Read the model definition and answer for the solid it produces. Units are mm, in the model's axes. Face numbers are marked on the shaded views. A direction names the side the tool comes from. Give positions to 0.01 mm unless a question says otherwise; leave off trailing zeros. Write each loop counter-clockwise with the first axis right and the second up, starting at its lowest first coordinate (ties: lowest second). Pieces come first, ordered by that corner, then holes. Notation, with made-up numbers: (38.5, 19.5) -> (58.5, 19.5) arc R10 cw to (58.5, 38.5) -> close; hole circle Ø11 at (-16.75, 22.25). An arc over 180 degrees is marked (long way). Use a Markdown table: item, result.
from build123d import *

# Parameters (mm, degrees)
EXTRUDE_THIN1_DEPTH     = 31.75
CUT_EXTRUDE1_DEPTH      = 79.232951004
CUT_EXTRUDE1_DEPTH_BACK = 79.232951004
SKETCH2_R               = 4.7625
SKETCH3_R               = 3.175
CUT_EXTRUDE2_DEPTH      = 56.93322439
FILLET1_R               = 9.525


with BuildPart() as part:
    # Sketch1 → Extrude-Thin1 (new, symmetric)
    with BuildSketch(Plane(origin=(0, 0, 0), x_dir=(0, 0, -1), z_dir=(1, 0, 0))):
        Polygon((0, 19.05), (0, 0), (-7.385338648, -15.83790984), (-10.372239485, -44.256373), (-12.721499107, -44.009455864), (-9.693278511, -15.19786147), (-2.3622, 0.523687132), (-2.3622, 19.05), align=None)
    extrude(amount=EXTRUDE_THIN1_DEPTH, both=True)

    # Sketch2 → Cut-Extrude1 (cut, two sides: drawn at the far end of the back side and taken through both)
    with BuildSketch(Plane(origin=(0, -51.169527341, 13.474052944), x_dir=(-1, 0, 0), z_dir=(0, 0.10452846326765357, 0.9945218953682734)).offset(-CUT_EXTRUDE1_DEPTH_BACK)):
        with Locations(Location((0, -26.249511152, 0), (0, 0, 270))):
            Circle(SKETCH2_R)
    extrude(amount=CUT_EXTRUDE1_DEPTH + CUT_EXTRUDE1_DEPTH_BACK, mode=Mode.SUBTRACT)

    # Sketch3 → Cut-Extrude2 (cut, through all)
    with BuildSketch(Plane(origin=(0, 0, 0), x_dir=(-1, 0, 0), z_dir=(0, 0, -1))):
        with Locations(Location((-22.225, 9.525, 0), (0, 0, 90))):
            Circle(SKETCH3_R)
        with Locations(Location((22.225, 9.525, 0), (0, 0, 90))):
            Circle(SKETCH3_R)
    extrude(amount=-CUT_EXTRUDE2_DEPTH, mode=Mode.SUBTRACT)

    # Fillet1
    fillet1_edges = [part.edges().sort_by_distance(p)[0] for p in [
        (31.75, 19.05, 1.1811),
        (-31.75, 19.05, 1.1811),
        (31.75, -44.132914432, 11.546869296),
        (-31.75, -44.132914432, 11.546869296),
    ]]
    fillet(fillet1_edges, radius=FILLET1_R)


solid = part.part
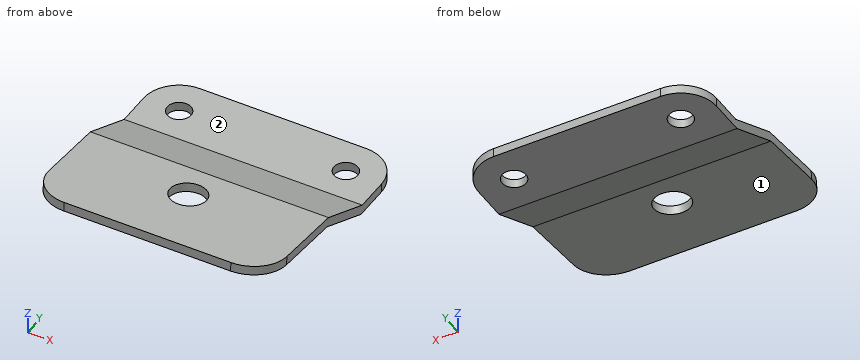
Item 1: A cutting plane is placed at D-D (x = 24.5). Give the vertices of the cut face in (y, z), then the cut area to 3 significant figures.
Return value:
| item | result |
|---|---|
| outline | (-43.98, 10.34) -> (-15.84, 7.39) -> (0, 0) -> (7.31, 0) -> (7.31, 2.36) -> (0.52, 2.36) -> (-15.2, 9.69) -> (-43.74, 12.69) -> close; (11.74, 0) -> (18.77, 0) -> (18.77, 2.36) -> (11.74, 2.36) -> close |
| area | 142 mm^2 |
Item 2: Straight lines are drawn through the part: line 1 along Z through (x, y) = (-8, 5); line 2 along X through (y, z) = (-28, 11); line 3 along Y through (x, z) = (-22, 1.5). For each, find the intervals that lie inside material, in ascending order. Write a range as [from, to].
Return value:
| item | result |
|---|---|
| line 1 | [0, 2.36] |
| line 2 | [-31.75, -3.74], [3.74, 31.75] |
| line 3 | [-3.22, 6.36], [12.69, 19.05] |
Item 3: A tool of negligible diameter and unlimited length cuts with its end or side. For the marked faces 1 and 2, from which of +Z, -Z, +X, -X, +Y, -Y can it reach the whole face along a straight path? Write none if from no direction.
Return value:
| item | result |
|---|---|
| face 1 | -Z, +X, -X, -Y |
| face 2 | +Z, +X, -X, +Y |
Item 4: A cutting plane is placed at C-C (x = -14.5). Give the vertices of the cut face in (y, z), then the cut area to 3 significant figures.
Return value:
| item | result |
|---|---|
| outline | (-44.26, 10.37) -> (-15.84, 7.39) -> (0, 0) -> (19.05, 0) -> (19.05, 2.36) -> (0.52, 2.36) -> (-15.2, 9.69) -> (-44.01, 12.72) -> close |
| area | 153 mm^2 |
Item 5: A cutting plane is placed at B-B (z = 1). Count the separate pieces of the cut face and the enclosed holes in it, then the cut area to 3 significant figures.
Return value:
| item | result |
|---|---|
| separate pieces | 1 |
| enclosed holes | 2 |
| area | 1,240 mm^2 |
Item 6: A cutting plane is placed at A-A (x = 3). Give the vertices of the cut face in (y, z), then the cut area to 3 significant figures.
Return value:
| item | result |
|---|---|
| outline | (-44.26, 10.37) -> (-28.99, 8.77) -> (-28.74, 11.12) -> (-44.01, 12.72) -> close; (-21.63, 7.99) -> (-15.84, 7.39) -> (0, 0) -> (19.05, 0) -> (19.05, 2.36) -> (0.52, 2.36) -> (-15.2, 9.69) -> (-21.39, 10.34) -> close |
| area | 136 mm^2 |
Item 7: Each of these flat-tipped pins is pushed along its axis until it touches: P1, Ø7.5, axis at x = -22.225, y = 9.525, coming from the -Z side; P2, Ø2, axis at x = 10.5, y = -26.5, coming from the +Z side; P3, Ø15, axis at x = 2, y = 7.5, coming from the +Z side; P4, Ø5, axis at x = -24.5, z = 10, coming from the +Y side. Where does it stop, or does it pass through?
Return value:
| item | result |
|---|---|
| P1 | z = 0 |
| P2 | z = 10.99 |
| P3 | z = 2.61 |
| P4 | y = -10.49 |
